Geometry: final body of the model. Coordinates: model frame, mm. Face numbers are marked on the shaded views. A direction names the side the tool comes from. Round coordinates to 2 decimals unless told otherwise and drop trailing zeros. Loops run counter-clockwise (first coordinate to the right, second up) from the corner with the lowest first, then second, coordinate; pieces in that order, holes last. Notation, with made-up numbers: (26, 52) - (33, 52) arc R21 ccw to (33, 91) - close; hole circle Ø8 at (17, 43.5). An arc over 180 degrees is marked (long way). Return JSON: item names as keys, results as strings. Group by question number.
1. Material intervals for probe 1 along Z at (x, y) = (0, -48); probe 2 along X at (y, z) = (-47.55, 0); probe 3 along Z at (x, y) = (0, -43), sorted ascending.
2. Section C-C on y = 12.5. Return loops of the section in (x, z).
3. Section A-A on y = -42. Return loops of the section in (x, z), and give its area (3 significant figures).
4. Set-up query: the marked faces 1 and 2. Return all of +Z, -Z, +X, -X, +Y, -Y with unobstructed straight access to the full face (end or side cutting, diameter ignored); none if empty.
5. Section B-B on y = -20. Return loops of the section in (x, z), and give its area (3 significant figures).
6. First-contact query: pin 1 Ø1 at (x, y) = (12.5, -29) entering from -Z; pin 2 Ø6 at (y, z) = (-11.5, -12.5) entering from +X; pin 3 Ø8 at (x, z) = (1, 2) entering from -Y; pin 4 Ø1 at (y, z) = (-2, 0) entering from +X. Flat tips, straight axial feed; report the tip coordinate or a pass-through.
7. Draft query along Z for the marked faces 3, 4 and 5. Return one class per face: +Z half, -Z half, draft (parallel to the pull), parting line (faces both ways), or undercut.
Autodesk Inventor part; units mm, degrees
sketch "Sketch1" plane through (0, 0, 0) normal (1, 0, 0) x (0, 1, 0)
  line L0 (20, 20) -> (-50, 20)
  line L1 (-50, 20) -> (-50, -20)
  line L2 (-50, -20) -> (20, -20)
  line L3 (20, -20) -> (20, 20)
  line L4 (-64, 0) -> (34, 0)
  line L5 (0, 28) -> (0, -28)
  line L6 (-50, 5) -> (-45, 5)
  line L7 (-45, 5) -> (-45, -5)
  line L8 (-45, -5) -> (-50, -5)
  line L9 (-50, -5) -> (-50, 5)
  line L10 (-45, 2.5) -> (-40, 2.5)
  line L11 (-40, 2.5) -> (-40, -2.5)
  line L12 (-40, -2.5) -> (-45, -2.5)
  line L13 (-45, -2.5) -> (-45, 2.5)
  line L14 (20, 0) -> (-9.519, 11.7284)
  line L15 (-9.519, 11.7284) -> (-9.519, 5)
  line L16 (20, 0) -> (-50, 0)
  line L17 (-9.519, 9.4368) -> (-23.459, 14.9754)
  line L18 (-23.459, 14.9754) -> (-23.459, 5)
  line L19 (-23.459, 12.5046) -> (-37.399, 18.0432)
  line L20 (-37.399, 18.0432) -> (-37.399, 5)
  line L21 (-37.399, 15.2739) -> (-50, 20)
  point P0 (0, 0)
  point P1 (-45, 0)
  point P2 (-40, 0)
  point P3 (0, 5)
  point P4 (0, 2.5)
  point P5 (0, 7.9463)
  dimension "d0" = 70
  dimension "d1" = 40
  dimension "d2" = 20
  dimension "d3" = 5
  dimension "d4" = 10
  dimension "d5" = 5
  dimension "d6" = 5
  dimension "d8" = 15
  dimension "d9" = 15
revolve "Revolution2" add sketch "Sketch1" angle 360 about axis through (0, 20, 0) along (0, -1, 0) contours L4 L5 L14 | L21 L20 L19 L18 L17 L15 L14 L5 L4 L11 L10 L7 L6 L1
properties part number "Tree_Leaves"
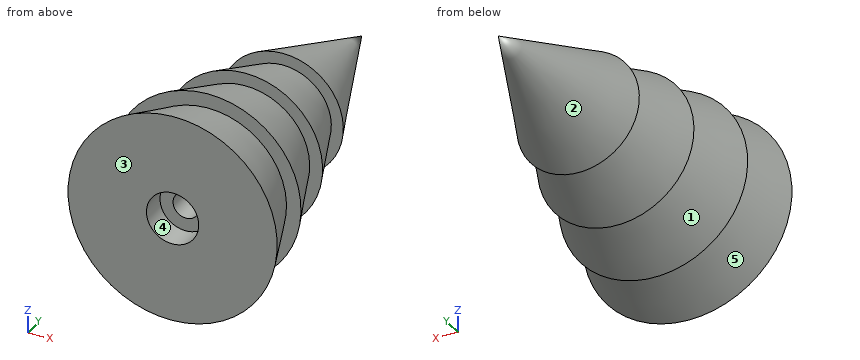
Taken from the geometry:
{
 "1": {"probe 1": "-19.25 to -5, 5 to 19.25", "probe 2": "-19.08 to -5, 5 to 19.08", "probe 3": "-17.37 to -2.5, 2.5 to 17.37"},
 "2": {"outline": "circle Ø5.96 at (0, 0)"},
 "3": {"outline": "circle Ø34 at (0, 0); hole circle Ø5 at (0, 0)", "area": "888 mm2"},
 "4": {"face 1": "none", "face 2": "+Y"},
 "5": {"outline": "circle Ø27.2 at (0, 0)", "area": "581 mm2"},
 "6": {"pin 1": "z = -8.58", "pin 2": "x = 5.71", "pin 3": "y = -50", "pin 4": "x = 8.94"},
 "7": {"face 3": "draft", "face 4": "undercut", "face 5": "parting line"}
}
